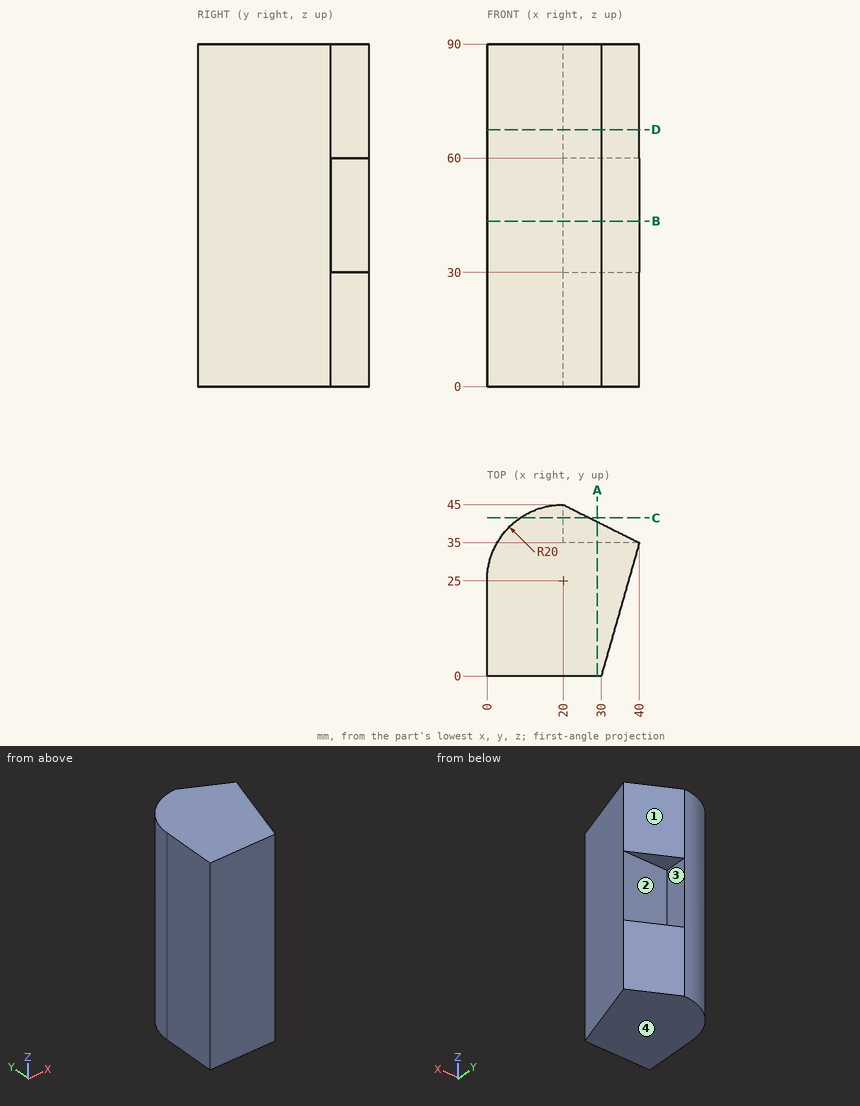
Design review of the part shown in the three views and the two pictorial views. Dimensions are in mm from the part's minimum x, y and z. Round coordinates to 2 decimals unless told otherwise and drop trailing zeros. Write each loop counter-clockwise with the first axis right and the second up, starting at its lowest first coordinate (ties: lowest second). Pieces come first, ordered by that corner, then holes.
1) Mouldability with a two-part tool opening along Z and no side actions: class the marked faces 1, 2, 3 and 4 as +Z half, -Z half, draft (parallel to the pull), parting line (faces both ways), or undercut.
Answer below:
face 1: draft
face 2: undercut
face 3: undercut
face 4: -Z half
2) Take a section at B-B on z = 43.5. Give the boundary of the cut face in (x, y).
Answer below:
outline: (0, 0) - (30, 0) - (40, 35) - (20, 35) - (20, 45) arc R20 ccw to (0, 25) - close
3) For line 1 along X through (y, z) = (4, 43); line 2 along X through (y, z) = (27, 76); line 3 along Y through (x, z) = (16.5, 44), list the stretches that pass through material, from the lowest coordinate up.
Answer below:
line 1: x = 0 to 31.14
line 2: x = 0.1 to 37.71
line 3: y = 0 to 44.69
4) Take a section at D-D on z = 67.5. Give the boundary of the cut face in (x, y).
Answer below:
outline: (0, 0) - (30, 0) - (40, 35) - (20, 45) arc R20 ccw to (0, 25) - close
5) Take a section at C-C on y = 41.5. Give the boundary of the cut face in (x, z).
Answer below:
outline: (8.7, 0) - (27, 0) - (27, 30) - (20, 30) - (20, 60) - (27, 60) - (27, 90) - (8.7, 90) - close
6) Take a section at A-A on x = 29. Give the boundary of the cut face in (y, z), then the cut area to 3 significant figures.
Answer below:
outline: (0, 0) - (40.5, 0) - (40.5, 30) - (35, 30) - (35, 60) - (40.5, 60) - (40.5, 90) - (0, 90) - close
area: 3,480 mm2
7) Insertion check: pin 1 Ø5 at (y, z) = (23.5, 36.5) entering from +X; pin 2 Ø2 at (y, z) = (22.5, 61.5) entering from +X; pin 3 Ø16 at (x, z) = (28.5, 49) entering from +Y. Each pin has a flat end and moves straight along its axis. Give the tip position at first contact, or say it passes through.
Answer below:
pin 1: stops at x = 37.43
pin 2: stops at x = 36.71
pin 3: stops at y = 35
